Could you check a few things on this model? Use its own coordinates, in mm. Face numbers are marked on the shaded views. A direction names the side the tool comes from. Give positions to 0.01 mm unless a question says otherwise; leave off trailing zeros. Write each loop counter-clockwise with the first axis right and the second up, starting at its lowest first coordinate (ties: lowest second). Pieces come first, ordered by that corner, then holes. Notation, with made-up numbers: (-1.75, 21.25) - (34.25, 21.25) arc R19 ccw to (34.25, 47.25) - close; hole circle Ø3 at (87.5, 19.5). An arc over 180 degrees is marked (long way). Answer as CSV lines item,"result". Start each with the question number.
Q1. On a 3-axis mill with a long thin cutter (end or side, diameter ignored), from which of +Z, -Z, +X, -X, +Y, -Y can I reach the whole of each face in a straight line? I mean the marked faces 4, 5 and 6. Say none if no direction works.
Q2. If I drill on line 1 along X through (y, z) = (1, 0); line 2 along X through (y, z) = (10.75, 0); line 3 along Y through (x, z) = (9, -2.25), over which ranges is the centre line in solid material (lowest first)?
Q3. Imagine slicing it at B-B on z = 0. List the corners of the cut face in (x, y) for me.
Q4. Imagine slicing it at D-D on z = 1.25. List the corners of the cut face in (x, y) for me, and give its area (3 significant figures).
Q5. Imagine slicing it at C-C on x = 7. List the corners of the cut face in (y, z) for me.
Q6. We'd pull the mould along X, two halves only. Please class the marked faces 1, 2 and 3: pulls with the +X half, pulls with the -X half, needs draft (parallel to the pull), parting line crosses it, or undercut.
Q7. Imagine slicing it at A-A on x = -8. List the corners of the cut face in (y, z) for me, and give its area (3 significant figures).
Q8. Will this pin go through, and if not, where does the flat tip stop? pin 1 Ø1.5 at (x, z) = (-7.5, -1) entering from -Y.
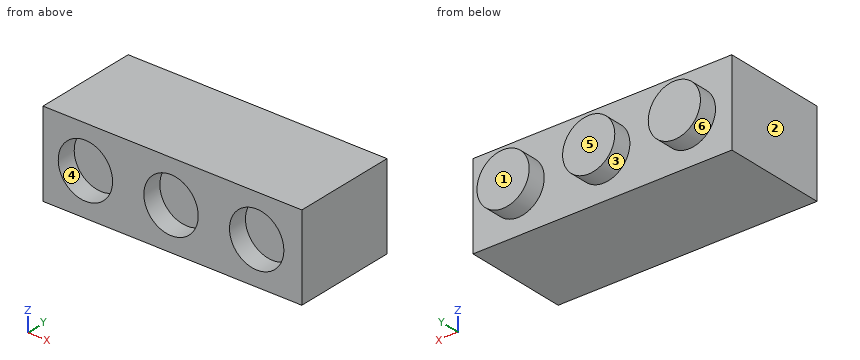
```python
from build123d import *

# Parameters (mm, degrees)
SKETCH_1_W          = 23.8
SKETCH_1_H          = 7.8
EXTRUDE_2_DEPTH     = 9.6
SKETCH_3_R          = 2.4
EXTRUDE_3_DEPTH     = 1.7
SKETCH_4_R          = 2.5
CUT_EXTRUDE_1_DEPTH = 1.8


with BuildPart() as part:
    # Эскиз1 → Бобышка-Вытянуть2 (new body)
    with BuildSketch(Plane(origin=(0, 0, 0), x_dir=(1, 0, 0), z_dir=(0, 1, 0))):
        Rectangle(SKETCH_1_W, SKETCH_1_H)
    extrude(amount=EXTRUDE_2_DEPTH)

    # Эскиз3 → Бобышка-Вытянуть3 (add)
    with BuildSketch(Plane(origin=(0, 9.6, 0), x_dir=(1, 0, 0), z_dir=(0, 1, 0))):
        with Locations(Location((-8, 0, 0), (0, 0, 270))):
            Circle(SKETCH_3_R)
        with Locations(Location((-0.126, 0, 0), (0, 0, 270))):
            Circle(SKETCH_3_R)
        with Locations(Location((7.748, 0, 0), (0, 0, 270))):
            Circle(SKETCH_3_R)
    extrude(amount=EXTRUDE_3_DEPTH)

    # Эскиз4 → Вырез-Вытянуть1 (cut)
    with BuildSketch(Plane.XZ):
        with Locations(Location((-8, 0, 0), (0, 0, 270))):
            Circle(SKETCH_4_R)
        with Locations(Location((-0.126, 0, 0), (0, 0, 270))):
            Circle(SKETCH_4_R)
        with Locations(Location((7.748, 0, 0), (0, 0, 270))):
            Circle(SKETCH_4_R)
    extrude(amount=-CUT_EXTRUDE_1_DEPTH, mode=Mode.SUBTRACT)


solid = part.part
```
Conclusion:
1,face 4,"-Y"
1,face 5,"+Z, -Z, +X, -X, +Y"
1,face 6,"+Y"
2,line 1,"-11.9 to -10.5, -5.5 to -2.63, 2.37 to 5.25, 10.25 to 11.9"
2,line 2,"-10.4 to -5.6, -2.53 to 2.27, 5.35 to 10.15"
2,line 3,"0 to 9.6"
3,outline,"(-11.9, 0) - (-10.5, 0) - (-10.5, 1.8) - (-5.5, 1.8) - (-5.5, 0) - (-2.63, 0) - (-2.63, 1.8) - (2.37, 1.8) - (2.37, 0) - (5.25, 0) - (5.25, 1.8) - (10.25, 1.8) - (10.25, 0) - (11.9, 0) - (11.9, 9.6) - (10.15, 9.6) - (10.15, 11.3) - (5.35, 11.3) - (5.35, 9.6) - (2.27, 9.6) - (2.27, 11.3) - (-2.53, 11.3) - (-2.53, 9.6) - (-5.6, 9.6) - (-5.6, 11.3) - (-10.4, 11.3) - (-10.4, 9.6) - (-11.9, 9.6) - close"
4,outline,"(-11.9, 0) - (-10.17, 0) - (-10.17, 1.8) - (-5.83, 1.8) - (-5.83, 0) - (-2.29, 0) - (-2.29, 1.8) - (2.04, 1.8) - (2.04, 0) - (5.58, 0) - (5.58, 1.8) - (9.91, 1.8) - (9.91, 0) - (11.9, 0) - (11.9, 9.6) - (9.8, 9.6) - (9.8, 11.3) - (5.7, 11.3) - (5.7, 9.6) - (1.92, 9.6) - (1.92, 11.3) - (-2.17, 11.3) - (-2.17, 9.6) - (-5.95, 9.6) - (-5.95, 11.3) - (-10.05, 11.3) - (-10.05, 9.6) - (-11.9, 9.6) - close"
4,area,"226 mm^2"
5,outline,"(0, -3.9) - (9.6, -3.9) - (9.6, -2.28) - (11.3, -2.28) - (11.3, 2.28) - (9.6, 2.28) - (9.6, 3.9) - (0, 3.9) - (0, 2.39) - (1.8, 2.39) - (1.8, -2.39) - (0, -2.39) - close"
6,face 1,"needs draft"
6,face 2,"pulls with the -X half"
6,face 3,"undercut"
7,outline,"(0, -3.9) - (9.6, -3.9) - (9.6, -2.4) - (11.3, -2.4) - (11.3, 2.4) - (9.6, 2.4) - (9.6, 3.9) - (0, 3.9) - (0, 2.5) - (1.8, 2.5) - (1.8, -2.5) - (0, -2.5) - close"
7,area,"74.0 mm^2"
8,pin 1,"y = 1.8"
